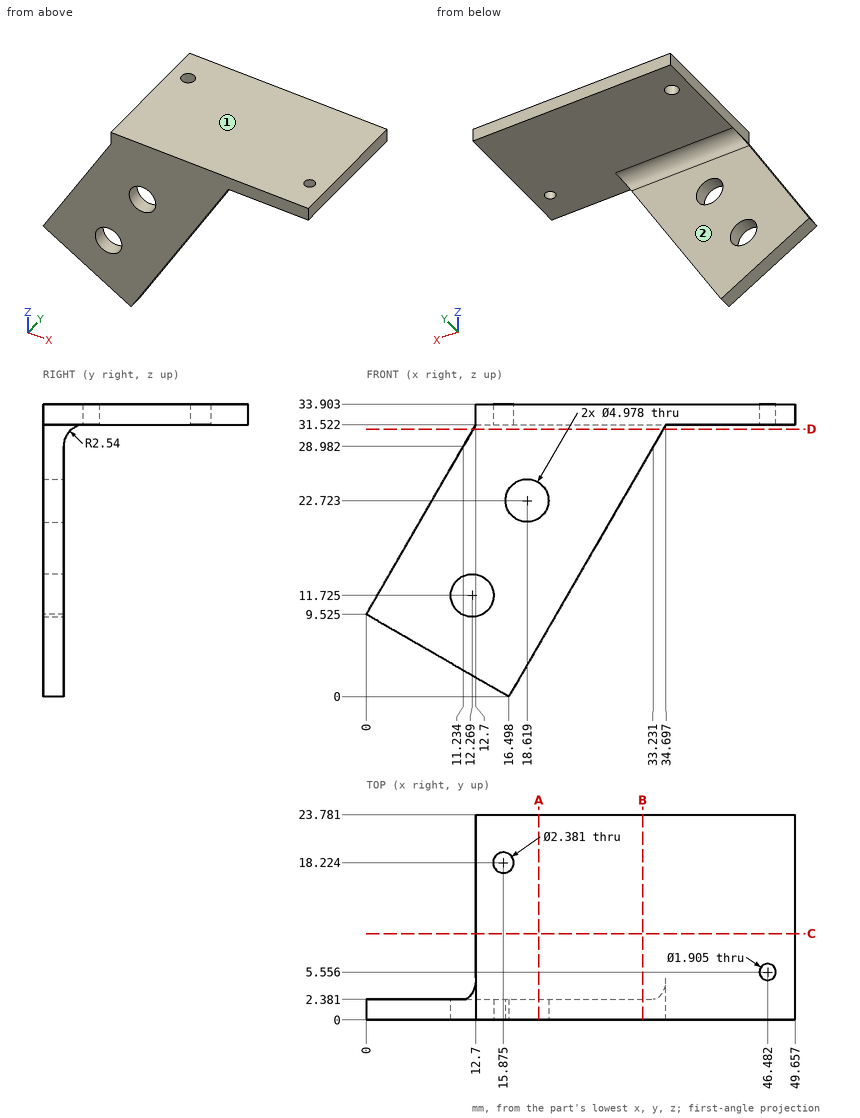
Could you check a few things on this drawing? It's one solid part, dimensions in mm from its lowest x, y, z. A direction names the side the tool comes from. Coordinates: 2 decimals unless noted, no trailing zeros. Order: outer loops, then holes, each group sorted by start corner. A loop starts at its lowest first (then second) coordinate and runs counter-clockwise, first axis right, second up.
1. If we section it at C-C (y = 10): Please give me the cut outline in (x, z).
2. I need wall thicknesses on line 1 (Y direction, x = 27.5, z = 25); line 2 (Z direction, x = 35.5, y = 6.25); line 3 (Z direction, x = 14, y = 2.25) (1 decimal). Which ranges of each line are inside material? Lowest first, please.
3. I'm going to push flat-ended pins straight in: pin 1 (2 mm diameter, centred on x = 23, z = 27.5, fed in from -Y); pin 2 (3 mm diameter, centred on x = 30, y = 16, fed in from -Z); pin 3 (2.5 mm diameter, centred on y = 13.5, z = 32.5, fed in from -X); pin 4 (5 mm diameter, centred on y = 4.5, z = 14.5, fed in from +X) (1 decimal). Where does each tip first touch, or does it pass through?
4. If we section it at B-B (x = 32): Please give me the cut outline in (y, z).
5. For the marked faces 1 and 2, which set-ups out of +Z, -Z, +X, -X, +Y, -Y let a thin tool reach every point of the face, with its end or its side?
6. If we section it at A-A (x = 20): Please give me the cut outline in (y, z).
7. If we section it at D-D (z = 31): Please give me the cut outline in (x, y) (1 decimal).
Entries:
1. outline: (12.7, 31.52) - (49.66, 31.52) - (49.66, 33.9) - (12.7, 33.9) - close
2. line 1: y = 0 to 2.38
2. line 2: z = 31.52 to 33.9
2. line 3: z = 1.4 to 9.9, 13.5 to 33.9
3. pin 1: stops at y = 0
3. pin 2: stops at z = 31.52
3. pin 3: stops at x = 12.7
3. pin 4: stops at x = 25.6
4. outline: (0, 26.85) - (2.38, 26.85) - (2.38, 28.98) arc R2.54 cw to (4.92, 31.52) - (23.78, 31.52) - (23.78, 33.9) - (0, 33.9) - close
5. face 1: +Z, +X, -X, +Y, -Y
5. face 2: -Z, +X, -X, +Y
6. outline: (0, 6.07) - (2.38, 6.07) - (2.38, 20.65) - (0, 20.65) - close; (0, 24.79) - (2.38, 24.79) - (2.38, 28.98) arc R2.54 cw to (4.92, 31.52) - (23.78, 31.52) - (23.78, 33.9) - (0, 33.9) - close
7. outline: (12.4, 0) - (34.4, 0) - (34.4, 3.4) - (12.4, 3.4) - close
